from build123d import *

# Parameters (mm, degrees)
SKETCH2_W           = 279.4
SKETCH2_H           = 279.4
SKETCH2_W_2         = 44.45
SKETCH2_H_2         = 5.5118
SKETCH2_W_3         = 5.5118
SKETCH2_H_3         = 44.45
BOSS_EXTRUDE1_DEPTH = 6.35


with BuildPart() as part:
    # Sketch2 → Boss-Extrude1 (new body)
    with BuildSketch(Plane.XY):
        Rectangle(SKETCH2_W, SKETCH2_H)
        with BuildLine():
            Line((-43.779617638, 39.738502384), (-120.083686649, 116.042571394))
            Line((-120.083686649, 116.042571394), (-116.042571394, 120.083686649))
            Line((-116.042571394, 120.083686649), (-39.738502384, 43.779617638))
            ThreePointArc((-39.738502384, 43.779617638), (-27.398923769, 36.969883512), (-13.328721415, 37.786636231))
            ThreePointArc((-13.328721415, 37.786636231), (0, 40.0685), (13.328721415, 37.786636231))
            ThreePointArc((13.328721415, 37.786636231), (27.398923769, 36.969883512), (39.738502384, 43.779617638))
            Line((39.738502384, 43.779617638), (116.042571394, 120.083686649))
            Line((116.042571394, 120.083686649), (120.083686649, 116.042571394))
            Line((120.083686649, 116.042571394), (43.779617638, 39.738502384))
            ThreePointArc((43.779617638, 39.738502384), (36.969883512, 27.398923769), (37.786636231, 13.328721415))
            ThreePointArc((37.786636231, 13.328721415), (40.0685, 0), (37.786636231, -13.328721415))
            ThreePointArc((37.786636231, -13.328721415), (36.969883512, -27.398923769), (43.779617638, -39.738502384))
            Line((43.779617638, -39.738502384), (120.083686649, -116.042571394))
            Line((120.083686649, -116.042571394), (116.042571394, -120.083686649))
            Line((116.042571394, -120.083686649), (39.738502384, -43.779617638))
            ThreePointArc((39.738502384, -43.779617638), (27.398923769, -36.969883512), (13.328721415, -37.786636231))
            ThreePointArc((13.328721415, -37.786636231), (0, -40.0685), (-13.328721415, -37.786636231))
            ThreePointArc((-13.328721415, -37.786636231), (-27.398923769, -36.969883512), (-39.738502384, -43.779617638))
            Line((-39.738502384, -43.779617638), (-116.042571394, -120.083686649))
            Line((-116.042571394, -120.083686649), (-120.083686649, -116.042571394))
            Line((-120.083686649, -116.042571394), (-43.779617638, -39.738502384))
            ThreePointArc((-43.779617638, -39.738502384), (-36.969883512, -27.398923769), (-37.786636231, -13.328721415))
            ThreePointArc((-37.786636231, -13.328721415), (-40.0685, 0), (-37.786636231, 13.328721415))
            ThreePointArc((-37.786636231, 13.328721415), (-36.969883512, 27.398923769), (-43.779617638, 39.738502384))
        make_face(mode=Mode.SUBTRACT)
        with Locations((0, -107.95)):
            Rectangle(SKETCH2_W_2, SKETCH2_H_2, mode=Mode.SUBTRACT)
        with Locations((-107.95, 0)):
            Rectangle(SKETCH2_W_3, SKETCH2_H_3, mode=Mode.SUBTRACT)
        with Locations((0, 107.95)):
            Rectangle(SKETCH2_W_2, SKETCH2_H_2, mode=Mode.SUBTRACT)
        with Locations((107.95, 0)):
            Rectangle(SKETCH2_W_3, SKETCH2_H_3, mode=Mode.SUBTRACT)
    extrude(amount=BOSS_EXTRUDE1_DEPTH)


solid = part.part
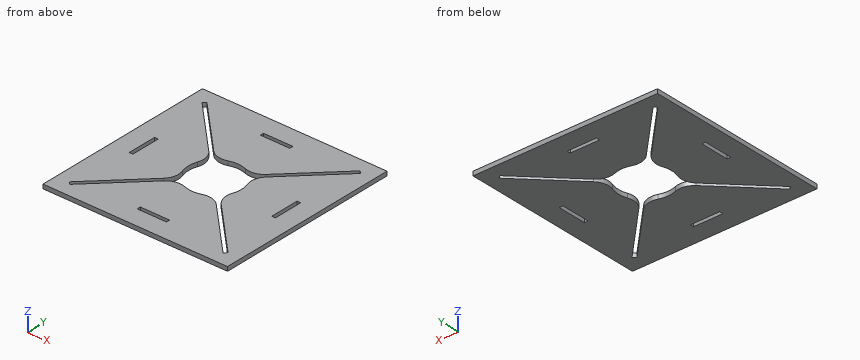
The model under review builds one solid part; all positions refer to its coordinate system, in mm. Round coordinates to 2 decimals unless told otherwise and drop trailing zeros. Order: outer loops, then holes, each group sorted by start corner. A loop starts at its lowest first (then second) coordinate and runs counter-clockwise, first axis right, second up. Notation, with made-up numbers: (63, 76) -> (82, 76) arc R19 cw to (82, 91) -> close; hole circle Ø6 at (58.25, 32.25). An arc over 180 degrees is marked (long way). Write item = value, one per line. Start each with the question number.
Item 1: Consider section A-A on y = 9. Write out the cut boundary in (x, z).
Item 2: For line 1 along X through (y, z) = (1, 4.75); line 2 along X through (y, z) = (-13.5, 5.5); line 3 along Y through (x, z) = (-96, 2), list the stretches that pass through material, from the lowest coordinate up.
Item 3: Consider section B-B on x = -58.5. Write out the cut boundary in (y, z), plus the area to 3 significant figures.
Item 4: Consider section D-D on z = 2.75. Count the separate pieces of the cut face and the enclosed holes in it, plus the area to 3 significant figures.
Item 5: Consider section C-C on y = -50.5. Write out the cut boundary in (x, z), plus the area to 3 significant figures.
Conclusion:
q1.outline = (-139.7, 0) -> (-110.71, 0) -> (-110.71, 6.35) -> (-139.7, 6.35) -> close; (-105.19, 0) -> (-39.04, 0) -> (-39.04, 6.35) -> (-105.19, 6.35) -> close; (39.04, 0) -> (105.19, 0) -> (105.19, 6.35) -> (39.04, 6.35) -> close; (110.71, 0) -> (139.7, 0) -> (139.7, 6.35) -> (110.71, 6.35) -> close
q2.line_1 = -139.7 to -110.71, -105.19 to -40.06, 40.06 to 105.19, 110.71 to 139.7
q2.line_2 = -139.7 to -110.71, -105.19 to -37.73, 37.73 to 105.19, 110.71 to 139.7
q2.line_3 = -139.7 to -100.04, -91.96 to 91.96, 100.04 to 139.7
q3.outline = (-139.7, 0) -> (-62.54, 0) -> (-62.54, 6.35) -> (-139.7, 6.35) -> close; (-54.46, 0) -> (54.46, 0) -> (54.46, 6.35) -> (-54.46, 6.35) -> close; (62.54, 0) -> (139.7, 0) -> (139.7, 6.35) -> (62.54, 6.35) -> close
q3.area = 1,670 mm2
q4.separate_pieces = 1
q4.enclosed_holes = 5
q4.area = 68,700 mm2
q5.outline = (-139.7, 0) -> (-54.54, 0) -> (-54.54, 6.35) -> (-139.7, 6.35) -> close; (-46.46, 0) -> (46.46, 0) -> (46.46, 6.35) -> (-46.46, 6.35) -> close; (54.54, 0) -> (139.7, 0) -> (139.7, 6.35) -> (54.54, 6.35) -> close
q5.area = 1,670 mm2
